from build123d import *

# Parameters (mm, degrees)
SKETCH_1_R               = 55
EXTRUDE_4_DEPTH          = 60
EXTRUDE_5_DEPTH          = 65
EXTRUDE_5_DEPTH_BACK     = 90
SKETCH_7_R               = 55
SKETCH_8_R               = 35
CUT_EXTRUDE_1_DEPTH      = 176.071414
SKETCH_10_R              = 60
EXTRUDE_6_DEPTH          = 12
SKETCH_11_R              = 35
CUT_EXTRUDE_3_DEPTH      = 20
PATTERN_CIRCULAR_1_COUNT = 10
SKETCH_14_R              = 50
CUT_EXTRUDE_4_DEPTH      = 20
SKETCH_16_R              = 47.5
CUT_EXTRUDE_5_DEPTH      = 25
PATTERN_CIRCULAR_2_COUNT = 12
SKETCH_19_R              = 51
CUT_EXTRUDE_6_DEPTH      = 63
SKETCH_21_R              = 42.49
CUT_EXTRUDE_7_DEPTH      = 57
PATTERN_CIRCULAR_3_COUNT = 12
CUT_EXTRUDE_8_DEPTH      = 130.938446966
CUT_EXTRUDE_8_DEPTH_BACK = 130.938446966
SKETCH_25_R              = 1
CUT_EXTRUDE_9_DEPTH      = 26
SKETCH_26_R              = 1
CUT_EXTRUDE_10_DEPTH     = 46
SKETCH_27_R              = 1
CUT_EXTRUDE_11_DEPTH     = 7
SKETCH_28_R              = 15
CUT_EXTRUDE_13_DEPTH     = 20


with BuildPart() as part:
    # 草图1 → 凸台-拉伸4 (new body)
    with BuildSketch(Plane.XY):
        Circle(SKETCH_1_R)
    extrude(amount=EXTRUDE_4_DEPTH)

    # 草图7 → 凸台-拉伸5 (add, two sides: drawn at the far end of the back side and taken through both)
    with BuildSketch(Plane(origin=(0, 0, 0), x_dir=(1, 0, 0), z_dir=(0, 1, 0)).offset(-EXTRUDE_5_DEPTH_BACK)):
        with Locations(Location((0, 0, 0), (0, 0, 270))):
            Circle(SKETCH_7_R)
    extrude(amount=EXTRUDE_5_DEPTH + EXTRUDE_5_DEPTH_BACK)

    # 草图8 → 切除-拉伸1 (cut, through all)
    with BuildSketch(Plane(origin=(0, 65, 0), x_dir=(1, 0, 0), z_dir=(0, 1, 0))):
        with Locations(Location((0, 0, 0), (0, 0, 270))):
            Circle(SKETCH_8_R)
    extrude(amount=-CUT_EXTRUDE_1_DEPTH, mode=Mode.SUBTRACT)

    # 草图10 → 凸台-拉伸6 (add)
    with BuildSketch(Plane.XY.offset(60)):
        Circle(SKETCH_10_R)
    extrude(amount=EXTRUDE_6_DEPTH)

    # 草图11 → 切除-拉伸3 (cut)
    with BuildSketch(Plane.XY.offset(72)):
        Circle(SKETCH_11_R)
    extrude(amount=-CUT_EXTRUDE_3_DEPTH, mode=Mode.SUBTRACT)

    # 草图12 → M4 螺纹孔1 (revolve, cut)
    with BuildSketch(Plane(origin=(0, 55, 72), x_dir=(0, -1, 0), z_dir=(1, 0, 0))):
        Polygon((0, 0), (0, 11.091420021), (1.65, 10.1), (1.65, 0), align=None)
    hole_wizard_m4_1 = revolve(axis=Axis((0, 55, 78.35), (0, 0, -1)), mode=Mode.SUBTRACT)

    # 阵列(圆周)1: M4 螺纹孔1 ×10 about axis
    pattern_circular_1_axis = Axis((0, 0, 0), (0, 0, 1))
    for i in range(1, PATTERN_CIRCULAR_1_COUNT):
        add(hole_wizard_m4_1.rotate(pattern_circular_1_axis, i * 360 / PATTERN_CIRCULAR_1_COUNT), mode=Mode.SUBTRACT)

    # 草图14 → 切除-拉伸4 (cut)
    with BuildSketch(Plane.XY.offset(72)):
        Circle(SKETCH_14_R)
    extrude(amount=-CUT_EXTRUDE_4_DEPTH, mode=Mode.SUBTRACT)

    # 草图16 → 切除-拉伸5 (cut)
    with BuildSketch(Plane.XZ.offset(90)):
        with Locations(Location((0, 0, 0), (0, 0, 270))):
            Circle(SKETCH_16_R)
    extrude(amount=-CUT_EXTRUDE_5_DEPTH, mode=Mode.SUBTRACT)

    # 草图17 → M3 螺纹孔1 (revolve, cut)
    with BuildSketch(Plane(origin=(0, -65, 42), x_dir=(0, 0, -1), z_dir=(1, 0, 0))):
        Polygon((0, 0), (0, 8.251075774), (1.25, 7.5), (1.25, 0), align=None)
    hole_wizard_m3_1 = revolve(axis=Axis((0, -71.35, 42), (0, 1, 0)), mode=Mode.SUBTRACT)

    # 阵列(圆周)2: M3 螺纹孔1 ×12 about axis
    pattern_circular_2_axis = Axis((0, 0, 0), (0, 1, 0))
    for i in range(1, PATTERN_CIRCULAR_2_COUNT):
        add(hole_wizard_m3_1.rotate(pattern_circular_2_axis, i * 360 / PATTERN_CIRCULAR_2_COUNT), mode=Mode.SUBTRACT)

    # 草图19 → 切除-拉伸6 (cut)
    with BuildSketch(Plane(origin=(0, 65, 0), x_dir=(1, 0, 0), z_dir=(0, 1, 0))):
        with Locations(Location((0, 0, 0), (0, 0, 270))):
            Circle(SKETCH_19_R)
    extrude(amount=-CUT_EXTRUDE_6_DEPTH, mode=Mode.SUBTRACT)

    # 草图21 → 切除-拉伸7 (cut)
    with BuildSketch(Plane(origin=(0, 2, 0), x_dir=(1, 0, 0), z_dir=(0, 1, 0))):
        with Locations(Location((0, 0, 0), (0, 0, 270))):
            Circle(SKETCH_21_R)
    extrude(amount=-CUT_EXTRUDE_7_DEPTH, mode=Mode.SUBTRACT)

    # 草图22 → M3 螺纹孔2 (revolve, cut)
    with BuildSketch(Plane(origin=(0, 2, -46.75), x_dir=(0, 0, 1), z_dir=(1, 0, 0))):
        Polygon((0, 0), (0, 8.251075774), (1.25, 7.5), (1.25, 0), align=None)
    hole_wizard_m3_2 = revolve(axis=Axis((0, 8.35, -46.75), (0, -1, 0)), mode=Mode.SUBTRACT)

    # 阵列(圆周)3: M3 螺纹孔2 ×12 about axis
    pattern_circular_3_axis = Axis((0, 0, 0), (0, 1, 0))
    for i in range(1, PATTERN_CIRCULAR_3_COUNT):
        add(hole_wizard_m3_2.rotate(pattern_circular_3_axis, i * 360 / PATTERN_CIRCULAR_3_COUNT), mode=Mode.SUBTRACT)

    # 草图24 → 切除-拉伸8 (cut, two sides: drawn at the far end of the back side and taken through both)
    with BuildSketch(Plane(origin=(0, 0, 0), x_dir=(0, 0, -1), z_dir=(1, 0, 0)).offset(-CUT_EXTRUDE_8_DEPTH_BACK)):
        Polygon((-55, 65), (55, 65), (55, 24.963274231), align=None)
    extrude(amount=CUT_EXTRUDE_8_DEPTH + CUT_EXTRUDE_8_DEPTH_BACK, mode=Mode.SUBTRACT)

    # 草图25 → 切除-拉伸9 (cut)
    with BuildSketch(Plane(origin=(0, 65, 0), x_dir=(1, 0, 0), z_dir=(0, 1, 0))):
        with Locations(Location((53, 0, 0), (0, 0, 270))):
            Circle(SKETCH_25_R)
        with Locations(Location((-53, 0, 0), (0, 0, 270))):
            Circle(SKETCH_25_R)
    extrude(amount=-CUT_EXTRUDE_9_DEPTH, mode=Mode.SUBTRACT)

    # 草图26 → 切除-拉伸10 (cut)
    with BuildSketch(Plane(origin=(0, 65, 0), x_dir=(1, 0, 0), z_dir=(0, 1, 0))):
        with Locations(Location((0, 53, 0), (0, 0, 270))):
            Circle(SKETCH_26_R)
    extrude(amount=-CUT_EXTRUDE_10_DEPTH, mode=Mode.SUBTRACT)

    # 草图27 → 切除-拉伸11 (cut)
    with BuildSketch(Plane(origin=(0, 65, 0), x_dir=(1, 0, 0), z_dir=(0, 1, 0))):
        with Locations(Location((0, -53, 0), (0, 0, 270))):
            Circle(SKETCH_27_R)
    extrude(amount=-CUT_EXTRUDE_11_DEPTH, mode=Mode.SUBTRACT)

    # 草图28 → 切除-拉伸13 (cut)
    with BuildSketch(Plane.XY.offset(52)):
        with Locations((0, 34)):
            Circle(SKETCH_28_R)
    extrude(amount=-CUT_EXTRUDE_13_DEPTH, mode=Mode.SUBTRACT)


solid = part.part
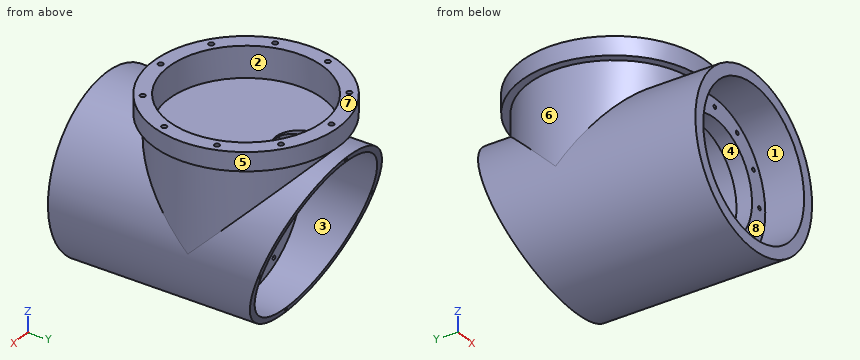
Geometry: final body of the model. Coordinates: model frame, mm. Face numbers are marked on the shaded views. A direction names the side the tool comes from. Round coordinates to 2 decimals unless told otherwise and drop trailing zeros. Order: outer loops, then holes, each group sorted by start corner. A loop starts at its lowest first (then second) coordinate and runs counter-clockwise, first axis right, second up.
Q1. Access query for the marked faces 1, 2, 3 and 4. Directions: +Z, -Z, +X, -X, +Y, -Y. A direction counts if a zero-diameter tool reaches every point of the face in a straight line with its end or side. Return the directions, or none.
Result sheet:
face 1: -Y
face 2: +Z
face 3: +Y
face 4: +Y, -Y
Q2. Pin query (flat end, axial travel): pin 1 (2 mm diameter, centred on x = 36.37, z = 21, fed in from +Y); pin 2 (4.5 mm diameter, centred on x = 32.33, y = -44.5, fed in from -Z); pin 3 (1 mm diameter, centred on x = -18, y = -70.5, fed in from -Z). Return the tip coordinate at first contact, or that it passes through.
Result sheet:
pin 1: stops at y = 2
pin 2: stops at z = -46.05
pin 3: stops at z = -52.14
Q3. Section A-A, the plane y = 10.5. Output: boundary loops of the cut face in (x, z), and give its area (3 significant figures).
Result sheet:
outline: (-59.07, 60) - (-53.99, 60) - (-53.99, 10.5) arc R55 ccw (long way) to (53.99, 10.5) - (53.99, 60) - (59.07, 60) - (59.07, 72) - (48.89, 72) - (48.89, 52) - (-48.89, 52) - (-48.89, 72) - (-59.07, 72) - close; hole circle Ø102 at (0, 0)
area: 2,540 mm2
Q4. Material intervals for probe 1 along X at (y, z) = (41, 0); probe 2 along X at (y, z) = (-63.25, -21); probe 3 along X at (y, z) = (-81.5, 0), sorted ascending.
Result sheet:
probe 1: x = -55 to -54, -52 to -51, 51 to 52, 54 to 55
probe 2: x = -50.83 to -37.62, -35.12 to -28, 28 to 35.12, 37.62 to 50.83
probe 3: x = -55 to -47.5, 47.5 to 55
Q5. Section B-B, the plane z = -27.5. Output: boundary loops of the cut face in (x, y), and give its area (3 significant figures).
Result sheet:
outline: (-47.63, -90) - (-38.73, -90) - (-38.73, -65) - (-21.65, -65) - (-21.65, -55) - (-32.39, -55) - (-32.39, 2) - (-42.95, 2) - (-42.95, 34.97) - (-47.63, 34.97) - close; (21.65, -65) - (38.73, -65) - (38.73, -90) - (47.63, -90) - (47.63, 34.97) - (42.95, 34.97) - (42.95, 2) - (32.39, 2) - (32.39, -55) - (21.65, -55) - close
area: 3,010 mm2
Q6. Mould query, pull axis Z, two halves, no side actions, for the marked faces 5, 6, 7 and 8. Classes: released by +Z, released by -Z, zero draft, split by the parting line, or undercut.
Result sheet:
face 5: zero draft
face 6: undercut
face 7: released by +Z
face 8: undercut
Q7. Section C-C, the plane z = -9. Output: boundary loops of the cut face in (x, y), and give its area (3 significant figures).
Result sheet:
outline: (-54.26, -90) - (-46.64, -90) - (-46.64, -65) - (-33.82, -65) - (-33.82, -55) - (-41.53, -55) - (-41.53, 2) - (-50.2, 2) - (-50.2, 41.71) - (-54.26, 41.71) - close; (33.82, -65) - (46.64, -65) - (46.64, -90) - (54.26, -90) - (54.26, 41.71) - (50.2, 41.71) - (50.2, 2) - (41.53, 2) - (41.53, -55) - (33.82, -55) - close
area: 2,560 mm2
Q8. Section D-D, the plane x = -6. Give the number of separate pieces and of enclosed holes in the cut face, and give its area (3 significant figures).
Result sheet:
separate pieces: 3
enclosed holes: 0
area: 2,560 mm2
